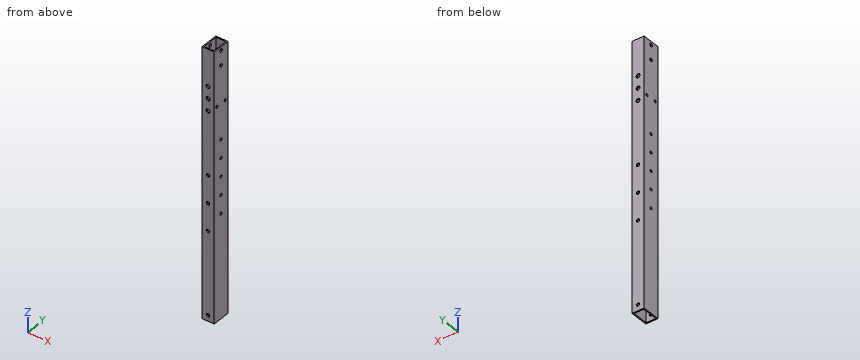
```python
from build123d import *

# Parameters (mm, degrees)
SKETCH1_W             = 10
SKETCH1_H             = 15
SKETCH1_W_2           = 8
SKETCH1_H_2           = 13
F_20_X_20_X_2_1_DEPTH = 12.5
SKETCH14_W            = 25
SKETCH14_H            = 15
SKETCH14_W_2          = 23
SKETCH14_H_2          = 13
F_20_X_20_X_2_8_DEPTH = 71
SKETCH_8_W            = 10
SKETCH_8_H            = 15
SKETCH_8_W_2          = 8
SKETCH_8_H_2          = 13
EXTRUDE_1_DEPTH       = 220
SKETCH_9_R            = 1.05
SKETCH_9_R_2          = 1.35
SKETCH_9_R_3          = 1.6
SKETCH_9_W            = 4
SKETCH_9_H            = 7
CUT_EXTRUDE_3_DEPTH   = 217.967739537
SKETCH_10_W           = 12
SKETCH_10_H           = 15
CUT_EXTRUDE_4_DEPTH   = 1
SKETCH_11_R           = 1.1
SKETCH_11_R_2         = 1.35
CUT_EXTRUDE_5_DEPTH   = 218.959285189
SKETCH_14_W           = 25
SKETCH_14_H           = 71
CUT_EXTRUDE_6_DEPTH   = 217.967739537


with BuildPart() as part:
    # Sketch1 → 方形管 20 X 20 X 2(1) (new body)
    with BuildSketch(Plane.ZY):
        Rectangle(SKETCH1_W, SKETCH1_H)
        Rectangle(SKETCH1_W_2, SKETCH1_H_2, mode=Mode.SUBTRACT)
    extrude(amount=F_20_X_20_X_2_1_DEPTH)


with BuildPart() as body_2:
    # Sketch14 → 方形管 20 X 20 X 2(8) (new body)
    with BuildSketch(Plane(origin=(-12.5, 0, -5), x_dir=(1, 0, 0), z_dir=(0, 0, 1))):
        Rectangle(SKETCH14_W, SKETCH14_H)
        Rectangle(SKETCH14_W_2, SKETCH14_H_2, mode=Mode.SUBTRACT)
    extrude(amount=F_20_X_20_X_2_8_DEPTH)


with BuildPart() as body_3:
    # 草图8 → 凸台-拉伸1 (new body)
    with BuildSketch(Plane.XY.offset(-5)):
        with Locations((5, 0)):
            Rectangle(SKETCH_8_W, SKETCH_8_H)
        with Locations((5, 0)):
            Rectangle(SKETCH_8_W_2, SKETCH_8_H_2, mode=Mode.SUBTRACT)
    extrude(amount=EXTRUDE_1_DEPTH)


with BuildPart() as cut_extrude_3_tool:
    # 草图9 → 切除-拉伸3 (new, through all)
    with BuildSketch(Plane(origin=(0, 7.5, 0), x_dir=(1, 0, 0), z_dir=(0, 1, 0))):
        with Locations(Location((-4, -48.5, 0), (0, 0, 270))):
            Circle(SKETCH_9_R)
        with Locations(Location((-21, -48.5, 0), (0, 0, 180))):
            Circle(SKETCH_9_R)
        with Locations(Location((-21, -12.5, 0), (0, 0, 270))):
            Circle(SKETCH_9_R)
        with Locations(Location((-4, -12.5, 0), (0, 0, 180))):
            Circle(SKETCH_9_R)
        with Locations(Location((-4.5, -61, 0), (0, 0, 270))):
            Circle(SKETCH_9_R_2)
        with Locations(Location((-20.5, -61, 0), (0, 0, 180))):
            Circle(SKETCH_9_R_2)
        with Locations(Location((5, -68, 0), (0, 0, 270))):
            Circle(SKETCH_9_R_2)
        with Locations(Location((5, -90.5, 0), (0, 0, 270))):
            Circle(SKETCH_9_R_2)
        with Locations(Location((5, -113, 0), (0, 0, 270))):
            Circle(SKETCH_9_R_2)
        with Locations(Location((5, -175, 0), (0, 0, 270))):
            Circle(SKETCH_9_R_3)
        with Locations(Location((-22, 0, 0), (0, 0, 270))):
            Circle(SKETCH_9_R_2)
        with Locations(Location((5, 0, 0), (0, 0, 270))):
            Circle(SKETCH_9_R_2)
        with Locations(Location((-3, 0, 0), (0, 0, 180))):
            Circle(SKETCH_9_R_2)
        with Locations(Location((5, -185, 0), (0, 0, 270))):
            Circle(SKETCH_9_R_3)
        with Locations((5, -165)):
            Circle(SKETCH_9_R_3)
        with Locations((-16.5, -15.5)):
            Rectangle(SKETCH_9_W, SKETCH_9_H)
        with Locations((-16.5, -45.5)):
            Rectangle(SKETCH_9_W, SKETCH_9_H)
        with Locations((-8.5, -45.5)):
            Rectangle(SKETCH_9_W, SKETCH_9_H)
        with Locations((-8.5, -15.5)):
            Rectangle(SKETCH_9_W, SKETCH_9_H)
    extrude(amount=-CUT_EXTRUDE_3_DEPTH)


with BuildPart() as part_1:
    add(part.part)

    # 切除-拉伸3: cut by cut_extrude_3_tool
    add(cut_extrude_3_tool.part, mode=Mode.SUBTRACT)


with BuildPart() as body_2_1:
    add(body_2.part)

    # 切除-拉伸3: cut by cut_extrude_3_tool
    add(cut_extrude_3_tool.part, mode=Mode.SUBTRACT)

    # 草图10 → 切除-拉伸4 (cut)
    with BuildSketch(Plane(origin=(0, 7.5, 0), x_dir=(1, 0, 0), z_dir=(0, 1, 0))):
        with Locations((-12.5, -30.5)):
            Rectangle(SKETCH_10_W, SKETCH_10_H)
    extrude(amount=-CUT_EXTRUDE_4_DEPTH, mode=Mode.SUBTRACT)

    # 草图14 → 切除-拉伸6 (cut, through all)
    with BuildSketch(Plane(origin=(0, 7.5, 0), x_dir=(1, 0, 0), z_dir=(0, 1, 0))):
        with Locations((-12.5, -30.5)):
            Rectangle(SKETCH_14_W, SKETCH_14_H)
    extrude(amount=-CUT_EXTRUDE_6_DEPTH, mode=Mode.SUBTRACT)


with BuildPart() as body_3_1:
    add(body_3.part)

    # 切除-拉伸3: cut by cut_extrude_3_tool
    add(cut_extrude_3_tool.part, mode=Mode.SUBTRACT)

    # 草图11 → 切除-拉伸5 (cut, through all)
    with BuildSketch(Plane(origin=(10, 0, 0), x_dir=(0, 0, -1), z_dir=(1, 0, 0))):
        with Locations((-80, 0)):
            Circle(SKETCH_11_R)
        with Locations((-95, 0)):
            Circle(SKETCH_11_R)
        with Locations((-110, 0)):
            Circle(SKETCH_11_R)
        with Locations((-125, 0)):
            Circle(SKETCH_11_R)
        with Locations((-140, 0)):
            Circle(SKETCH_11_R)
        with Locations((-212, 0)):
            Circle(SKETCH_11_R_2)
        with Locations((-200, 0)):
            Circle(SKETCH_11_R_2)
        with Locations((-169, -4.5)):
            Circle(SKETCH_11_R)
        with Locations((-169, 4.5)):
            Circle(SKETCH_11_R)
    extrude(amount=-CUT_EXTRUDE_5_DEPTH, mode=Mode.SUBTRACT)


solid = body_3_1.part
```
CAD build for the part. Positions are in the model's coordinates, mm. Round coordinates to 2 decimals unless told otherwise and drop trailing zeros. Order: outer loops, then holes, each group sorted by start corner. A loop starts at its lowest first (then second) coordinate and runs counter-clockwise, first axis right, second up. Notation, with made-up numbers: (76, 70) - (86, 70) arc R27 cw to (86, 97) - close; hole circle Ø11 at (54, 57.5). An arc over 180 degrees is marked (long way). Answer in a Markdown table with one row per item. Add a question column.
(1) Drop a flat-ended pin along its axis: pin 1 Ø3 at (y, z) = (0, 140) entering from -X. Give the stop position or say it passes through.
(2) Probe L1, parallel to X at y = -2.25, z = 59.5; L2, parallel to Y at x = 9.5, z = 95; L3, parallel to Y at x = 8, z = 98. List the from-to ranges inside material, lowest first. Write a range as [from, to].
(3) Band-saw the part on A-A on z = 33. List the corners of the cut face in (x, y), and give its area (3 significant figures).
Data:
| question | item | result |
|---|---|---|
| 1 | pin 1 | stops at x = 0 |
| 2 | L1 | x = [0, 1], [9, 10] |
| 2 | L2 | y = [-7.5, -1.1], [1.1, 7.5] |
| 2 | L3 | y = [-7.5, -6.5], [6.5, 7.5] |
| 3 | outline | (0, -7.5) - (10, -7.5) - (10, 7.5) - (0, 7.5) - close; hole (1, -6.5) - (9, -6.5) - (9, 6.5) - (1, 6.5) - close |
| 3 | area | 46.0 mm^2 |
